Input: dimensioned drawing with shaded views. Units: mm. Origin: part minimum x, y, z. A direction names the side the tool comes from. Round coordinates to 2 decimals unless told otherwise and drop trailing zeros. Loops run counter-clockwise (first coordinate to the right, second up) from the corner with the lowest first, then second, coordinate; pieces in that order, holes last. Notation, with made-up numbers: (8.25, -8) - (39.25, -8) arc R20 cw to (39.25, 0) - close; hole circle Ø8 at (-39, 84). An arc over 180 degrees is marked (long way). Write each question's results on one line, items separated by ' | '.
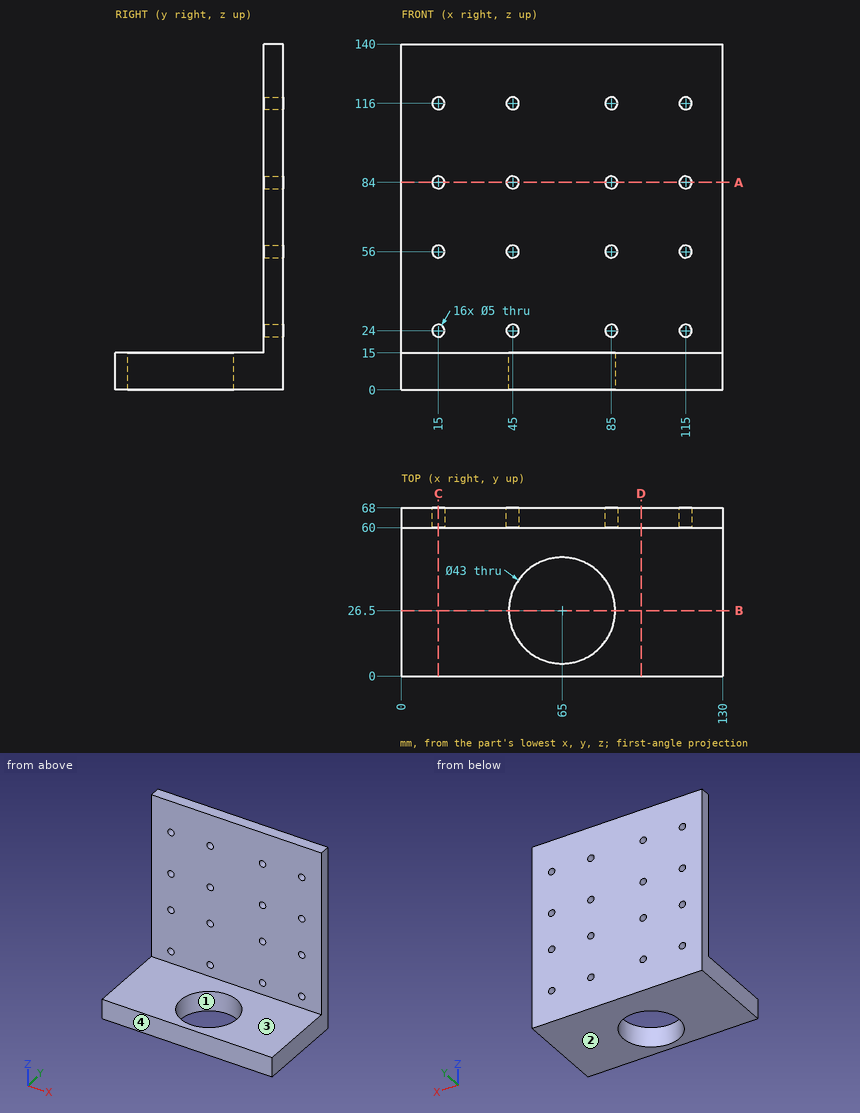
1. Section query C-C, the plane x = 15. Output: boundary loops of the cut face in (y, z), plus the area to 3 significant figures.
Answer:
outline: (0, 0) - (68, 0) - (68, 21.5) - (60, 21.5) - (60, 15) - (0, 15) - close; (60, 26.5) - (68, 26.5) - (68, 53.5) - (60, 53.5) - close; (60, 58.5) - (68, 58.5) - (68, 81.5) - (60, 81.5) - close; (60, 86.5) - (68, 86.5) - (68, 113.5) - (60, 113.5) - close; (60, 118.5) - (68, 118.5) - (68, 140) - (60, 140) - close | area: 1,860 mm^2
2. Mould query, pull axis X, two halves, no side actions, for the marked faces 1 and 2. Classes: pulls with the +X half, pulls with the -X half, needs draft (parallel to the pull), parting line crosses it, or undercut.
Answer:
face 1: undercut | face 2: needs draft
3. Line query: line 1 (Z direction, x = 85, y = 62.75); line 2 (Y direction, x = 65, z = 3); line 3 (Z direction, x = 122, y = 25). Output: solid intervals per line, ascending. Write a range as [from, to].
Answer:
line 1: [0, 21.5], [26.5, 53.5], [58.5, 81.5], [86.5, 113.5], [118.5, 140] | line 2: [0, 5], [48, 68] | line 3: [0, 15]
4. Section query D-D, the plane x = 97. Output: boundary loops of the cut face in (y, z).
Answer:
outline: (0, 0) - (68, 0) - (68, 140) - (60, 140) - (60, 15) - (0, 15) - close
5. Contact query for flat-ended pins moving along their axis: pin 1 (8 mm diameter, centred on x = 115, z = 84, fed in from -Y); pin 2 (12 mm diameter, centred on x = 21, y = 36, fed in from +Z); pin 3 (8 mm diameter, centred on x = 115, z = 56, fed in from +Y); pin 4 (3 mm diameter, centred on x = 45, z = 56, fed in from -Y). Output: stop coordinate, or through.
Answer:
pin 1: y = 60 | pin 2: z = 15 | pin 3: y = 68 | pin 4: through
6. Section query B-B, the plane y = 26.5. Output: boundary loops of the cut face in (x, z), plus the area to 4 significant figures.
Answer:
outline: (0, 0) - (43.5, 0) - (43.5, 15) - (0, 15) - close; (86.5, 0) - (130, 0) - (130, 15) - (86.5, 15) - close | area: 1,305 mm^2
7. Section query A-A, the plane z = 84. Output: boundary loops of the cut face in (x, y), plus the area to 3 significant figures.
Answer:
outline: (0, 60) - (12.5, 60) - (12.5, 68) - (0, 68) - close; (17.5, 60) - (42.5, 60) - (42.5, 68) - (17.5, 68) - close; (47.5, 60) - (82.5, 60) - (82.5, 68) - (47.5, 68) - close; (87.5, 60) - (112.5, 60) - (112.5, 68) - (87.5, 68) - close; (117.5, 60) - (130, 60) - (130, 68) - (117.5, 68) - close | area: 880 mm^2
8. Set-up query: the marked faces 3 and 4. Return all of +Z, -Z, +X, -X, +Y, -Y with unobstructed straight access to the full face (end or side cutting, diameter ignored); none if empty.
Answer:
face 3: +Z, +X, -X, -Y | face 4: +Z, -Z, +X, -X, -Y
